```python
from build123d import *

# Parameters (mm, degrees)
SKETCH_1_W      = 20
SKETCH_1_H      = 3
SKETCH_1_W_2    = 3
SKETCH_1_H_2    = 20
EXTRUDE_1_DEPTH = 3


with BuildPart() as part:
    # Эскиз1 → Бобышка-Вытянуть1 (new body)
    with BuildSketch(Plane.XY):
        Polygon((0, 0), (90, 0), (180, 0), (180, 20), (108, 20), (108, 28), (180, 28), (180, 72), (108, 72), (108, 80), (180, 80), (180, 100), (90, 100), (0, 100), (-90, 100), (-90, 80), (-18, 80), (-18, 72), (-90, 72), (-90, 28), (-18, 28), (-18, 20), (-90, 20), (-90, 0), align=None)
        with Locations((28, 4.5)):
            Rectangle(SKETCH_1_W, SKETCH_1_H, mode=Mode.SUBTRACT)
        with Locations((62, 95.5)):
            Rectangle(SKETCH_1_W, SKETCH_1_H, mode=Mode.SUBTRACT)
        with Locations((4.5, 35)):
            Rectangle(SKETCH_1_W_2, SKETCH_1_H_2, mode=Mode.SUBTRACT)
        with Locations((85.5, 65)):
            Rectangle(SKETCH_1_W_2, SKETCH_1_H_2, mode=Mode.SUBTRACT)
    extrude(amount=EXTRUDE_1_DEPTH)


solid = part.part
```
Geometry check sheet. Reference: the model listing, model coordinates, mm. Coordinates: 2 decimals unless noted, no trailing zeros. Write each loop counter-clockwise with the first axis right and the second up, starting at its lowest first coordinate (ties: lowest second). Pieces come first, ordered by that corner, then holes. Notation, with made-up numbers: M 57.25,-38 L 97.25,-38 A23 ccw 97.25,-26 Z; hole C 89.25,45.5 d2. An arc over 180 degrees is marked long. Answer as a JSON object with one key per item and string values.
1. Scan lines: L1, parallel to Y at x = 160, z = 2.85; L2, parallel to Y at x = 20, z = 2.7; L3, parallel to X at y = 40, z = 0.3. Record each from-to range of solid material in increasing order.
Answers below:
{"L1": "y = 0 to 20, 28 to 72, 80 to 100", "L2": "y = 0 to 3, 6 to 100", "L3": "x = -90 to 3, 6 to 180"}
2. Section check B-B, the plane z = 1.8. Give the number of separate pieces and of enclosed holes in the cut face, plus the area to 3 significant figures.
Answers below:
{"separate pieces": "1", "enclosed holes": "4", "area": "24,500 mm²"}
3. Section check A-A, the plane x = -35. Enter the section's corners in (y, z).
Answers below:
{"outline": "M 0,0 L 20,0 L 20,3 L 0,3 Z; M 28,0 L 72,0 L 72,3 L 28,3 Z; M 80,0 L 100,0 L 100,3 L 80,3 Z"}
